Design review of the part built by this model. Coordinates are the model's own, in mm. A direction names the side the tool comes from. Coordinates: 2 decimals unless noted, no trailing zeros. Loops run counter-clockwise (first coordinate to the right, second up) from the corner with the lowest first, then second, coordinate; pieces in that order, holes last. Notation, with made-up numbers: M -36.5,36 L -6.5,36 A20 ccw -6.5,44 Z; hole C 68,-28.5 d3. An arc over 180 degrees is marked long. One line per item, written item: value.
Autodesk Inventor part; units mm, degrees
ref_plane "YZ Plane" through (0, 0, 0) normal (1, 0, 0) x (0, 1, 0)
ref_plane "XZ Plane" through (0, 0, 0) normal (0, 1, 0) x (-1, 0, 0)
ref_plane "XY Plane" through (0, 0, 0) normal (0, 0, 1) x (1, 0, 0)
sketch "Sketch1" plane through (0, 0, 0) normal (0, 0, 1) x (1, 0, 0)
  line L0 (-155, 55) -> (155, 55)
  line L1 (155, 55) -> (155, -55)
  line L2 (155, -55) -> (-155, -55)
  line L3 (-155, -55) -> (-155, 55)
  point P0 (0, 0)
  dimension "d0" = 110
  dimension "d1" = 310
  dimension "d2" = 155
  dimension "d3" = 55
extrude "Extrusion1" add sketch "Sketch1" along normal blind 10
sketch "Sketch2" plane through (0, 0, 10) normal (0, 0, 1) x (1, 0, 0)
  line L0 (155, 55) -> (-155, 55)
  point P0 (0, 0)
  point P1 (-37.5, 44)
  point P2 (37.5, 44)
  point P3 (-37.5, -31)
  point P4 (37.5, -31)
  dimension "d6" = 75
  dimension "d7" = 11
  dimension "d8" = 75
  dimension "d27" = 37.5
hole "Hole1" at (-37.5, 44, 10) at (37.5, 44, 10) at (-37.5, -31, 10) at (37.5, -31, 10) direction (0, 0, -1) diameter 6.6 end through all counterbore diameter 11 counterbore depth 7
sketch "Sketch3" plane through (0, 0, 0) normal (0, 0, -1) x (-1, 0, 0)
  point P0 (0, 0)
  point P1 (-140, 40)
  point P2 (-140, -40)
  point P3 (140, 40)
  point P4 (140, -40)
  dimension "d16" = 80
  dimension "d17" = 40
  dimension "d18" = 280
  dimension "d19" = 140
hole "Hole2" at (140, 40, 0) at (140, -40, 0) at (-140, 40, 0) at (-140, -40, 0) direction (0, 0, 1) diameter 6.6 end through all counterbore diameter 11 counterbore depth 7
properties part number "zStagePostAttach"
(1) We need section B-B on x = 37.5. State the section outline as (y, z) points.
Reply:
outline: M -55,0 L -34.3,0 L -34.3,3 L -36.5,3 L -36.5,10 L -55,10 Z; M -27.7,0 L 40.7,0 L 40.7,3 L 38.5,3 L 38.5,10 L -25.5,10 L -25.5,3 L -27.7,3 Z; M 47.3,0 L 55,0 L 55,10 L 49.5,10 L 49.5,3 L 47.3,3 Z
(2) We need section A-A on y = -31. State the section outline as (x, z) points, then the cut area to 3 significant figures.
Reply:
outline: M -155,0 L -40.8,0 L -40.8,3 L -43,3 L -43,10 L -155,10 Z; M -34.2,0 L 34.2,0 L 34.2,3 L 32,3 L 32,10 L -32,10 L -32,3 L -34.2,3 Z; M 40.8,0 L 155,0 L 155,10 L 43,10 L 43,3 L 40.8,3 Z
area: 2,910 mm2
(3) Insertion check: pin 1 (9 mm diameter, centred on x = 140, y = -40, fed in from -Z); pin 2 (5.5 mm diameter, centred on x = -140, y = 40, fed in from +Z). Each pin has a flat end and moves straight along its axis. Give the tip position at first contact, or say it passes through.
Reply:
pin 1: stops at z = 7
pin 2: passes through
(4) Mouldability with a two-part tool opening along X and no side actions: class faces 1 (the flat face through (-2, 1, 0)), 2 (the cylindrical face through (-145.453, -40.716, 3.549)), 3 (the flat face through (-155, -1, 5)) as released by +X, released by -X, zero draft, split by the parting line, or undercut.
Reply:
face 1: zero draft
face 2: undercut
face 3: released by -X
(5) Tool access review of faces 4 (the cylindrical face through (143.22, 39.28, 8.52)), 5 (the flat face through (144, 40, 7)), 6 (the cylindrical face through (-41.22, -26.95, 6.45)): name each direction out of +Z, -Z, +X, -X, +Y, -Y from which nothing blocks a thin tool from reaching the whole face with its end or side.
Reply:
face 4: +Z, -Z
face 5: -Z
face 6: +Z
(6) To check wall thickness, follow line 1 along X through (y, z) = (40, 2.75); line 2 along Y through (x, z) = (37.5, 0.8); line 3 along Y through (x, z) = (-37.5, 7.25). State the ranges of each line that lie inside material, in increasing order. Write a range as [from, to].
Reply:
line 1: x = [-155, -145.5], [-134.5, 134.5], [145.5, 155]
line 2: y = [-55, -34.3], [-27.7, 40.7], [47.3, 55]
line 3: y = [-55, -36.5], [-25.5, 38.5], [49.5, 55]
